Autodesk Fusion 360 part; units mm, degrees
sketch "Sketch1" plane through (0, 0, 0) normal (0, 1, 0) x (1, 0, 0)
  line L0 (0, -150) -> (0, -65)
  line L1 (0, -65) -> (40, -65)
  line L2 (40, -65) -> (40, -100)
  line L3 (0, 0) -> (225, 0)
  line L4 (225, -40) -> (225, 0)
  line L5 (40, -100) -> (110, -100)
  line L6 (0, -150) -> (150, -150)
  line L7 (110, -100) -> (110, 0)
  line L8 (150, -150) -> (150, -40)
  line L9 (150, -40) -> (225, -40)
  dimension "d7" = 150
  dimension "d9" = 85
  dimension "d11" = 35
  dimension "d14" = 225
  dimension "d15" = 70
  dimension "d16" = 150
  dimension "d17" = 110
extrude "Extrude1" add sketch "Sketch1" along normal blind 200
sketch "Sketch2" plane through (0, 0, 0) normal (0, 0, 1) x (1, 0, 0)
  line L0 (224.8321, 0) -> (425, 0) construction
  line L1 (225, 200) -> (270, 200) construction
  line L2 (224.8321, 0) -> (269.8321, 0) construction
  line L3 (350, 145) -> (280, 145)
  line L4 (350.0871, 55.0001) -> (279.6959, 54.8638)
  line L5 (225, 200) -> (280, 145)
  line L6 (225, 200) -> (302.7817, 200) construction
  line L7 (224.8321, 0) -> (256.6519, 31.8198)
  line L8 (256.6519, 31.8198) -> (279.6959, 54.8638)
  arc A0 (350.0871, 55.0001) -> (350, 145) centre (350, 100) ccw
  line L9 (225, 200) -> (224.8321, 0)
  dimension "d24" = 90
  dimension "d29" = 45
  dimension "d30" = 45
extrude "Extrude2" add sketch "Sketch2" along normal blind 40
sketch "Sketch3" plane through (0, 0, 40) normal (0, 0, 1) x (-1, 0, 0)
  line L0 (-150, 0) -> (-225, 0)
  line L1 (-225, 0) -> (-225, -0.1679)
  line L2 (-225, -0.1679) -> (-279.6959, -54.8638)
  line L3 (-279.6959, -54.8638) -> (-350.0871, -55.0001)
  arc A0 (-350.0871, -55.0001) -> (-350, -145) centre (-350, -100) ccw
  line L4 (-350, -145) -> (-280, -145)
  line L5 (-280, -145) -> (-225, -200)
  line L6 (-225, -200) -> (-150, -200)
  line L7 (-150, -200) -> (-150, 0)
  circle A1 centre (-350, -100) radius 25
extrude "Extrude3" cut sketch "Sketch3" against normal blind 40 contours A1
sketch "Sketch4" plane through (0, 0, 150) normal (0, 0, 1) x (-1, 0, 0)
  line L0 (0, 0) -> (-150, 0)
  line L1 (-150, 0) -> (-150, -200)
  line L2 (-150, -200) -> (0, -200)
  line L3 (0, -200) -> (0, 0)
  circle A0 centre (-75, -155) radius 25
  circle A1 centre (-75, -45) radius 25
extrude "Extrude4" cut sketch "Sketch4" against normal blind 20 contours A0 | A1
sketch "Sketch5" plane through (0, 0, 150) normal (0, 0, 1) x (-1, 0, 0)
  circle A0 centre (-75, -155) radius 25
  circle A1 centre (-75, -45) radius 25
  line L0 (0, 0) -> (-150, 0)
  line L1 (-150, 0) -> (-150, -200)
  line L2 (-150, -200) -> (0, -200)
  line L3 (0, -200) -> (0, 0)
  circle A2 centre (-75, -155) radius 12.5
  circle A3 centre (-75, -45) radius 12.5
  dimension "d43" = 25
  dimension "d44" = 25
extrude "Extrude5" cut sketch "Sketch5" against normal blind 80 contours A2 | A3
extrude "Extrude6" add sketch "Sketch2" along normal blind 40
sketch "Sketch6" plane through (0, 0, 40) normal (0, 0, 1) x (-1, 0, 0)
  line L0 (-150, 0) -> (-225, 0)
  line L1 (-225, 0) -> (-225, -0.1679)
  line L2 (-225, -0.1679) -> (-279.6959, -54.8638)
  line L3 (-279.6959, -54.8638) -> (-350.0871, -55.0001)
  arc A0 (-350.0871, -55.0001) -> (-350, -145) centre (-350, -100) ccw
  line L4 (-350, -145) -> (-280, -145)
  line L5 (-280, -145) -> (-225, -200)
  line L6 (-225, -200) -> (-150, -200)
  line L7 (-150, -200) -> (-150, 0)
  circle A1 centre (-350, -100) radius 25
  dimension "d49" = 50
extrude "Extrude7" cut sketch "Sketch6" against normal blind 60 contours A1
Model file for the job. Use its own axes, mm. A direction names the side the tool comes from. Coordinates: 2 decimals unless noted, no trailing zeros. Order: outer loops, then holes, each group sorted by start corner. A loop starts at its lowest first (then second) coordinate and runs counter-clockwise, first axis right, second up. Notation, with made-up numbers: (-35, 8) - (-1, 8) arc R29 ccw to (-1, 29) - close; hole circle Ø9 at (45.25, 13.25). An arc over 180 degrees is marked (long way). Return JSON: item names as keys, results as strings. Group by question number.
1) Saw through at C-C, the plane x = 75. Write the cut outline in (y, z).
2) Flat gauge pins, fed straight in: P1, Ø10, axis at y = 85.5, z = 58, coming from the +X side; P2, Ø8, axis at x = 287, y = 149.5, coming from the -Z side; P3, Ø8, axis at x = 196, y = 68, coming from the +Z side; P4, Ø5, axis at y = 78, z = 85.5, coming from the -X side. Where does each tip first touch, or does it go through?
3) Saw through at D-D, the plane z = 14.5. Write the cut outline in (x, y), plus the area to 3 significant figures.
4) Tool access for faces 4 (the flat face through (315, 145, 20)), 5 (the flat face through (150, 99, 96)), 6 (the flat face through (75, 99, 100)), 7 (the cylindrical face through (78.255, 130.213, 140.14)), 8 (the flat face through (74, 99, 150)): list every direction of +Z, -Z, +X, -X, +Y, -Y with a clear straight run to the whole face (end or side of a thin tool).
5) Probe line 1 (Y direction, x = 75, z = 141.5); line 2 (X direction, y = 189, z = 91); line 3 (X direction, y = 45, z = 123). List the from-to ranges inside material, lowest first. Write a range as from..to.
6) Saw through at A-A, the plane y = 155. Write the cut outline in (x, z), plus the area to 4 significant figures.
7) Saw through at B-B, the plane z = 85. Write the cut outline in (x, y).
8) Mould opens along X. For faces 1 (the flat face through (20, 99, 65)), 2 (the flat face through (252, 173, 20)), 3 (the flat face through (110, 99, 51)) say: released by +X, released by -X, zero draft, split by the parting line, or undercut.
Values found:
{
 "1": {"outline": "(0, 100) - (32.5, 100) - (32.5, 130) - (20, 130) - (20, 150) - (0, 150) - close; (57.5, 100) - (142.5, 100) - (142.5, 130) - (130, 130) - (130, 150) - (70, 150) - (70, 130) - (57.5, 130) - close; (167.5, 100) - (200, 100) - (200, 150) - (180, 150) - (180, 130) - (167.5, 130) - close"},
 "2": {"P1": "stops at x = 150", "P2": "passes through", "P3": "stops at z = 40", "P4": "stops at x = 0"},
 "3": {"outline": "(110, 0) - (225, 0) - (225, 0.17) - (279.7, 54.86) - (350.09, 55) arc R45 ccw to (350, 145) - (280, 145) - (225, 200) - (110, 200) - close; hole circle Ø50 at (350, 100)", "area": "38,500 mm²"},
 "4": {"face 4": "+Z, -Z, +X, +Y", "face 5": "+Z, +X, +Y, -Y", "face 6": "-Z, +Y, -Y", "face 7": "+Z", "face 8": "+Z, +X, -X, +Y, -Y"},
 "5": {"line 1": "y = 0..20, 70..130, 180..200", "line 2": "x = 0..40, 110..150", "line 3": "x = 0..62.5, 87.5..150"},
 "6": {"outline": "(0, 65) - (40, 65) - (40, 100) - (62.5, 100) - (62.5, 130) - (50, 130) - (50, 150) - (0, 150) - close; (87.5, 100) - (110, 100) - (110, 0) - (270, 0) - (270, 40) - (150, 40) - (150, 150) - (100, 150) - (100, 130) - (87.5, 130) - close", "area": "15,950 mm²"},
 "7": {"outline": "(0, 0) - (40, 0) - (40, 200) - (0, 200) - close; (110, 0) - (150, 0) - (150, 200) - (110, 200) - close"},
 "8": {"face 1": "zero draft", "face 2": "released by +X", "face 3": "undercut"}
}
